Verification items for the finished model (mm, model axes). A direction names the side the tool comes from. Coordinates: 2 decimals unless noted, no trailing zeros. Order: outer loops, then holes, each group sorted by start corner. A loop starts at its lowest first (then second) coordinate and runs counter-clockwise, first axis right, second up. Notation, with made-up numbers: (25, 57.25) - (37, 57.25) arc R29 cw to (37, 85.25) - close; hole circle Ø9 at (-29, 49). An arc over 180 degrees is marked (long way). Answer as CSV lines item,"result". Start each with the question number.
1. Go/stop test with flat-tipped pins: pin 1 (4 mm diameter, centred on x = 63, y = 1.5, fed in from -Z); pin 2 (1 mm diameter, centred on x = 34, z = 1.5, fed in from +Y); pin 3 (0.9 mm diameter, centred on x = 67, z = 1, fed in from +Y); pin 4 (8 mm diameter, centred on x = 77.5, y = 10.5, fed in from -Z). Record where each tip stops, or that it passes through.
2. Material ranges on L1, parallel to X at y = 2.25, z = 4.75; L2, parallel to Y at x = 31, z = 3.25; L3, parallel to X at y = 5.75, z = 0, recorded low to high. Write a range as [from, to].
3. Section check B-B (y = 14.5). Count the separate pieces of the cut face and the enclosed holes in it, and give its area (3 significant figures).
4. Mould release check, pull along Y, two halves, no side actions. Record for faces 1 (the flat face through (118.8, -1.194, 0.686)), 2 (the flat face through (66.499, 15, 2)): pulls with the +Y half, pulls with the -Y half, needs draft (parallel to the pull), parting line crosses it, or undercut.
5. Set-up check for faces 3 (the flat face through (76, 9, 4.1)), 4 (the flat face through (-0.4, 10.2, -1.3)): record each of +Z, -Z, +X, -X, +Y, -Y from which the full face is reachable in a straight line by a thin tool's end or side.
6. Section check A-A (x = 51). Record the cut outline in (y, z).
from build123d import *

# Parameters (mm, degrees)
SKETCH005_W     = 122.986
SKETCH005_H     = 21.18
SKETCH005_W_2   = 119.986
SKETCH005_H_2   = 18.18
PAD004_DEPTH    = 9.9
SKETCH006_W     = 122.986
SKETCH006_H     = 21.18
PAD005_DEPTH    = 1.5
SKETCH007_W     = 13.9
SKETCH007_H     = 14.3
POCKET001_DEPTH = 9.901
SKETCH008_R     = 1.45
SKETCH008_W     = 1.5
SKETCH008_H     = 18.18
PAD006_DEPTH    = 3.5
SKETCH009_W     = 7
SKETCH009_H     = 2
SKETCH009_W_2   = 13
PAD007_DEPTH    = 2
POCKET002_DEPTH = 6.5
SKETCH011_W     = 99.287
SKETCH011_H     = 1.5
POCKET003_DEPTH = 6
SKETCH012_W     = 1.5
SKETCH012_H     = 21.18
POCKET004_DEPTH = 3
CHAMFER003_SIZE = 2
SKETCH013_W     = 2
SKETCH013_H     = 18.18
PAD008_DEPTH    = 3.5


with BuildPart() as part:
    # Sketch005 (on ShapeBinder) → Pad004 (new body)
    with BuildSketch(Plane(origin=(-93.484762, 101.426, -4.3), x_dir=(1, 0, 0), z_dir=(0, 0, -1))):
        with Locations((153.277762, 92.79)):
            Rectangle(SKETCH005_W, SKETCH005_H)
        with Locations((153.277762, 92.79)):
            Rectangle(SKETCH005_W_2, SKETCH005_H_2, mode=Mode.SUBTRACT)
    extrude(amount=-PAD004_DEPTH)

    # Sketch006 (on Face10 of Pad004) → Pad005 (join)
    with BuildSketch(Plane(origin=(-93.484762, 101.426, 5.6), x_dir=(1, 0, 0), z_dir=(0, 0, 1))):
        with Locations((153.277762, -92.79)):
            Rectangle(SKETCH006_W, SKETCH006_H)
    extrude(amount=-PAD005_DEPTH)

    # Sketch007 (on Face16 of Pad005) → Pocket001 (cut, through all)
    with BuildSketch(Plane(origin=(-93.484762, 101.426, 5.6), x_dir=(1, 0, 0), z_dir=(0, 0, 1))):
        with Locations((101.358762, -92.79)):
            Rectangle(SKETCH007_W, SKETCH007_H)
        with Locations((125.158762, -92.79)):
            Rectangle(SKETCH007_W, SKETCH007_H)
        with Locations((148.958762, -92.79)):
            Rectangle(SKETCH007_W, SKETCH007_H)
    extrude(amount=-POCKET001_DEPTH, mode=Mode.SUBTRACT)

    # Sketch008 (on Face15 of Pocket001) → Pad006 (join)
    with BuildSketch(Plane(origin=(-93.484762, 101.426, 4.1), x_dir=(1, 0, 0), z_dir=(0, 0, -1))):
        with BuildLine():
            Line((112.483762, 96.208699), (112.483762, 101.88))
            Line((112.483762, 101.88), (113.983762, 101.88))
            Line((113.983762, 101.88), (113.983762, 96.208699))
            ThreePointArc((113.983762, 89.371301), (116.733762, 92.79), (113.983762, 96.208699))
            Line((113.983762, 83.7), (113.983762, 89.371301))
            Line((112.483762, 83.7), (113.983762, 83.7))
            Line((112.483762, 83.7), (112.483762, 89.371301))
            ThreePointArc((112.483762, 96.208699), (109.733762, 92.79), (112.483762, 89.371301))
        make_face()
        with Locations((113.233762, 92.79)):
            Circle(SKETCH008_R, mode=Mode.SUBTRACT)
        with Locations((136.983762, 92.79)):
            Rectangle(SKETCH008_W, SKETCH008_H)
        with BuildLine():
            Line((159.983762, 101.88), (161.483762, 101.88))
            Line((161.483762, 101.88), (161.483762, 96.208699))
            ThreePointArc((161.483762, 89.371301), (164.233762, 92.79), (161.483762, 96.208699))
            Line((161.483762, 83.7), (161.483762, 89.371301))
            Line((159.983762, 83.7), (161.483762, 83.7))
            Line((159.983762, 83.7), (159.983762, 89.371301))
            ThreePointArc((159.983762, 96.208699), (157.233762, 92.79), (159.983762, 89.371301))
            Line((159.983762, 101.88), (159.983762, 96.208699))
        make_face()
        with Locations((160.733762, 92.79)):
            Circle(SKETCH008_R, mode=Mode.SUBTRACT)
    extrude(amount=PAD006_DEPTH)

    # Sketch009 (on Face27 of Pad006) → Pad007 (join)
    with BuildSketch(Plane(origin=(-93.484762, 101.426, 4.1), x_dir=(1, 0, 0), z_dir=(0, 0, -1))):
        with Locations((194.770762, 84.7)):
            Rectangle(SKETCH009_W, SKETCH009_H)
        with Locations((191.770762, 100.88)):
            Rectangle(SKETCH009_W_2, SKETCH009_H)
    extrude(amount=PAD007_DEPTH)

    # Sketch010 (on Face5 of Pad007) → Pocket002 (cut)
    with BuildSketch(Plane(origin=(121.286, 101.426, -1.6), x_dir=(0, 1, 0), z_dir=(1, 0, 0))):
        with BuildLine():
            ThreePointArc((-95.29, 6.7), (-97.04, 4.95), (-95.29, 3.2))
            Line((-95.29, 3.2), (-90.29, 3.2))
            ThreePointArc((-90.29, 3.2), (-88.54, 4.95), (-90.29, 6.7))
            Line((-95.29, 6.7), (-90.29, 6.7))
        make_face()
    extrude(amount=-POCKET002_DEPTH, mode=Mode.SUBTRACT)

    # Sketch011 (on Face2 of Pocket002) → Pocket003 (cut)
    with BuildSketch(Plane(origin=(-93.484762, 101.426, -4.3), x_dir=(1, 0, 0), z_dir=(0, 0, -1))):
        with Locations((163.627262, 102.63)):
            Rectangle(SKETCH011_W, SKETCH011_H)
        with Locations((163.627262, 82.95)):
            Rectangle(SKETCH011_W, SKETCH011_H)
    extrude(amount=-POCKET003_DEPTH, mode=Mode.SUBTRACT)

    # Sketch012 (on Face6 of Pocket003) → Pocket004 (cut)
    with BuildSketch(Plane(origin=(-93.484762, 101.426, -4.3), x_dir=(1, 0, 0), z_dir=(0, 0, -1))):
        Polygon((113.983762, 103.38), (113.983762, 101.88), (93.284762, 101.88), (93.284762, 83.7), (113.983762, 83.7), (113.983762, 82.2), (91.784762, 82.2), (91.784762, 103.38), align=None)
        with Locations((214.020762, 92.79)):
            Rectangle(SKETCH012_W, SKETCH012_H)
    extrude(amount=-POCKET004_DEPTH, mode=Mode.SUBTRACT)

    # Chamfer003
    chamfer003_edges = [part.edges().sort_by_distance(p)[0] for p in [
        (119.786, 18.476, 1.7),
        (119.786, -1.204, 1.7),
    ]]
    chamfer(chamfer003_edges, length=CHAMFER003_SIZE)

    # Sketch013 (on Face31 of Chamfer003) → Pad008 (join)
    with BuildSketch(Plane(origin=(-93.484762, 101.426, 4.1), x_dir=(1, 0, 0), z_dir=(0, 0, -1))):
        with Locations((178.950762, 92.79)):
            Rectangle(SKETCH013_W, SKETCH013_H)
    extrude(amount=PAD008_DEPTH)


solid = part.part
Evaluation:
1,pin 1,"stops at z = 1.7"
1,pin 2,"stops at y = 19.23"
1,pin 3,"stops at y = 17.73"
1,pin 4,"stops at z = 4.1"
2,L1,"x = [-1.7, 0.92], [14.82, 24.72], [38.62, 48.52], [62.42, 121.29]"
2,L2,"y = [-1.95, -0.45], [17.73, 19.23]"
2,L3,"x = [-1.7, -0.2], [119.79, 121.29]"
3,separate pieces,"4"
3,enclosed holes,"0"
3,area,"161 mm²"
4,face 1,"needs draft"
4,face 2,"undercut"
5,face 3,"-Z"
5,face 4,"-Z, +X, -X, +Y, -Y"
6,outline,"(-1.95, 1.7) - (-0.45, 1.7) - (-0.45, 4.1) - (1.49, 4.1) - (1.49, 5.6) - (-1.95, 5.6) - close; (15.79, 4.1) - (17.73, 4.1) - (17.73, 1.7) - (19.23, 1.7) - (19.23, 5.6) - (15.79, 5.6) - close"
